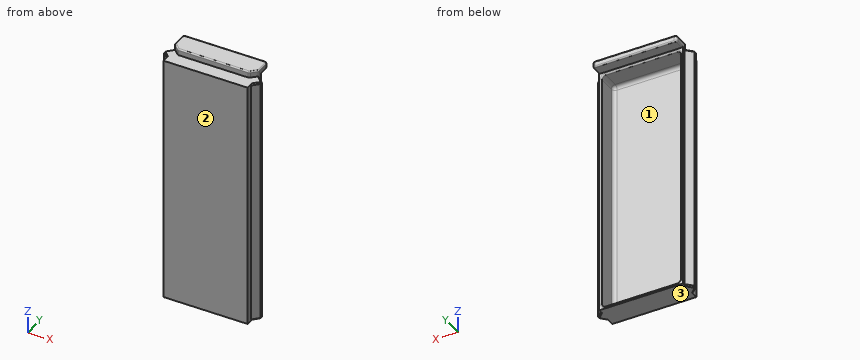
```python
from build123d import *

# Parameters (mm, degrees)
EXTRUDE_1_DEPTH     = 200
SKETCH_2_W          = 63
SKETCH_2_H          = 196
CUT_EXTRUDE_1_DEPTH = 17
SKETCH_3_W          = 67
SKETCH_3_H          = 17
EXTRUDE_2_DEPTH     = 5
CHAMFER_1_SIZE      = 5
FILLET_1_R          = 2
FILLET_2_R          = 1
FILLET_3_R          = 3
FILLET_4_R          = 1
CHAMFER_2_SIZE      = 1


with BuildPart() as part:
    # 草图1 → 凸台-拉伸1 (new body)
    with BuildSketch(Plane.XY):
        Polygon((-73, 28), (-6, 28), (-6, 32.656854249), (-1, 37.656854249), (-1, 39.353196257), (-6, 44.353196257), (-6, 47), (-73, 47), (-73, 44.353196257), (-78, 39.353196257), (-78, 37.656854249), (-73, 32.656854249), align=None)
    extrude(amount=-EXTRUDE_1_DEPTH)

    # 草图2 → 切除-拉伸1 (cut)
    with BuildSketch(Plane(origin=(0, 47, 0), x_dir=(1, 0, 0), z_dir=(0, 1, 0))):
        with Locations((-39.5, 100)):
            Rectangle(SKETCH_2_W, SKETCH_2_H)
    extrude(amount=-CUT_EXTRUDE_1_DEPTH, mode=Mode.SUBTRACT)

    # 草图3 → 凸台-拉伸2 (add)
    with BuildSketch(Plane.XY):
        with Locations((-39.5, 47.5)):
            Rectangle(SKETCH_3_W, SKETCH_3_H)
    extrude(amount=EXTRUDE_2_DEPTH)

    # 倒角1
    chamfer_1_edges = [part.edges().sort_by_distance(p)[0] for p in [
        (-73, 39, 2.5),
        (-6, 39, 2.5),
    ]]
    chamfer(chamfer_1_edges, length=CHAMFER_1_SIZE)

    # 圆角1
    fillet_1_edges = [part.edges().sort_by_distance(p)[0] for p in [
        (-6, 56, 2.5),
        (-6, 44, 2.5),
        (-11, 39, 2.5),
        (-68, 39, 2.5),
        (-73, 44, 2.5),
        (-73, 56, 2.5),
    ]]
    fillet(fillet_1_edges, radius=FILLET_1_R)

    # 圆角2
    fillet_2_edges = [part.edges().sort_by_distance(p)[0] for p in [
        (-6, 50.5, 0),
        (-39.5, 56, 0),
        (-39.5, 56, 5),
        (-73, 50.5, 0),
        (-72.414213562, 55.414213562, 0),
        (-6.585786438, 55.414213562, 0),
        (-6, 49.414213562, 5),
        (-39.5, 39, 5),
        (-8.5, 41.5, 5),
        (-73, 49.414213562, 5),
        (-70.5, 41.5, 5),
        (-72.414213562, 55.414213562, 5),
        (-72.847759065, 44.06306026, 5),
        (-67.93693974, 39.152240935, 5),
        (-11.06306026, 39.152240935, 5),
        (-6.152240935, 44.06306026, 5),
        (-6.585786438, 55.414213562, 5),
    ]]
    fillet(fillet_2_edges, radius=FILLET_2_R)

    # 圆角3
    fillet_3_edges = [part.edges().sort_by_distance(p)[0] for p in [
        (-39.5, 30, -2),
        (-8, 38.5, -2),
        (-8, 30, -100),
        (-8, 38.5, -198),
        (-39.5, 30, -198),
        (-71, 38.5, -198),
        (-71, 30, -100),
        (-71, 38.5, -2),
    ]]
    fillet(fillet_3_edges, radius=FILLET_3_R)

    # 圆角4
    fillet_4_edges = [part.edges().sort_by_distance(p)[0] for p in [
        (-39.5, 47, -198),
        (-8, 47, -100),
        (-39.5, 47, -2),
        (-71, 47, -100),
        (-8.878679656, 47, -2.878679656),
        (-8.878679656, 47, -197.121320344),
        (-70.121320344, 47, -2.878679656),
        (-70.121320344, 47, -197.121320344),
    ]]
    fillet(fillet_4_edges, radius=FILLET_4_R)

    # 倒角2
    chamfer_2_edges = [part.edges().sort_by_distance(p)[0] for p in [
        (-75.5, 35.156854249, 0),
        (-78, 38.505025253, 0),
        (-75.476752896, 41.876443361, 0),
        (-3.523247104, 41.876443361, 0),
        (-1, 38.505025253, 0),
        (-3.5, 35.156854249, 0),
        (-3.5, 35.156854249, -200),
        (-1, 38.505025253, -200),
        (-3.523247104, 41.876443361, -200),
        (-75.476752896, 41.876443361, -200),
        (-78, 38.505025253, -200),
        (-75.5, 35.156854249, -200),
    ]]
    chamfer(chamfer_2_edges, length=CHAMFER_2_SIZE)


solid = part.part
```
Geometry: final body of the model. Coordinates: model frame, mm. Face numbers are marked on the shaded views. Round coordinates to 2 decimals unless told otherwise and drop trailing zeros. Order: outer loops, then holes, each group sorted by start corner. A loop starts at its lowest first (then second) coordinate and runs counter-clockwise, first axis right, second up. Notation, with made-up numbers: (23, -12.5) -> (70, -12.5) arc R34 ccw to (70, 21.5) -> close; hole circle Ø8 at (-20, -16.75). An arc over 180 degrees is marked (long way). Write each question's results on one line, items separated by ' | '.
Q1. Section query B-B (z = -187). Output: boundary loops of the cut face in (x, y), and give its area (3 significant figures).
Response values:
outline: (-78, 37.66) -> (-73, 32.66) -> (-73, 28) -> (-6, 28) -> (-6, 32.66) -> (-1, 37.66) -> (-1, 39.35) -> (-6.05, 44.4) arc R2 ccw to (-6, 44.83) -> (-6, 47) -> (-7, 47) arc R1 ccw to (-8, 46) -> (-8, 33) arc R3 cw to (-11, 30) -> (-68, 30) arc R3 cw to (-71, 33) -> (-71, 46) arc R1 ccw to (-72, 47) -> (-73, 47) -> (-73, 44.83) arc R2 ccw to (-72.95, 44.4) -> (-78, 39.35) -> close | area: 272 mm²
Q2. Section query C-C (y = 52). Output: boundary loops of the cut face in (x, z), and give its area (3 significant figures).
Response values:
outline: (-73, 1) arc R1 ccw to (-72, 0) -> (-7, 0) arc R1 ccw to (-6, 1) -> (-6, 4) arc R1 ccw to (-7, 5) -> (-72, 5) arc R1 ccw to (-73, 4) -> close | area: 334 mm²
Q3. Pin query (flat end, axial travel): pin 1 Ø7.5 at (y, z) = (48.5, -48) entering from -X; pin 2 Ø10 at (y, z) = (48.5, -65.5) entering from +X; pin 3 Ø5 at (y, z) = (30.5, -66) entering from +X; pin 4 Ø3 at (y, z) = (37.5, -117) entering from +X. Return the tip coordinate at first contact, or that it passes through.
Response values:
pin 1: x = -73 | pin 2: x = -5.15 | pin 3: x = -5.66 | pin 4: x = -1
Q4. Pull-direction query (Z, two-part tool) for the marked faces 1, 2 and 3; classes: released by +Z, released by -Z, zero draft, split by the parting line, or undercut.
Response values:
face 1: undercut | face 2: zero draft | face 3: released by -Z
Q5. Ray query, line 1 along X through (y, z) = (45, -178.5); line 2 along Z through (x, y) = (-67.5, 41.5); line 3 along X through (y, z) = (38.5, -20). Return the intervals inside material, ascending.
Response values:
line 1: -73 to -71, -8 to -6 | line 2: -200 to -198, -2 to 5 | line 3: -78 to -71, -8 to -1
Q6. Section query A-A (x = -17.5). Output: boundary loops of the cut face in (y, z), and give its area (3 significant figures).
Response values:
outline: (28, -200) -> (47, -200) -> (47, -199) arc R1 ccw to (46, -198) -> (33, -198) arc R3 cw to (30, -195) -> (30, -5) arc R3 cw to (33, -2) -> (46, -2) arc R1 ccw to (47, -1) -> (47, 0) -> (55, 0) arc R1 ccw to (56, 1) -> (56, 4) arc R1 ccw to (55, 5) -> (40, 5) arc R1 ccw to (39, 4) -> (39, 0) -> (28, 0) -> close | area: 556 mm²
